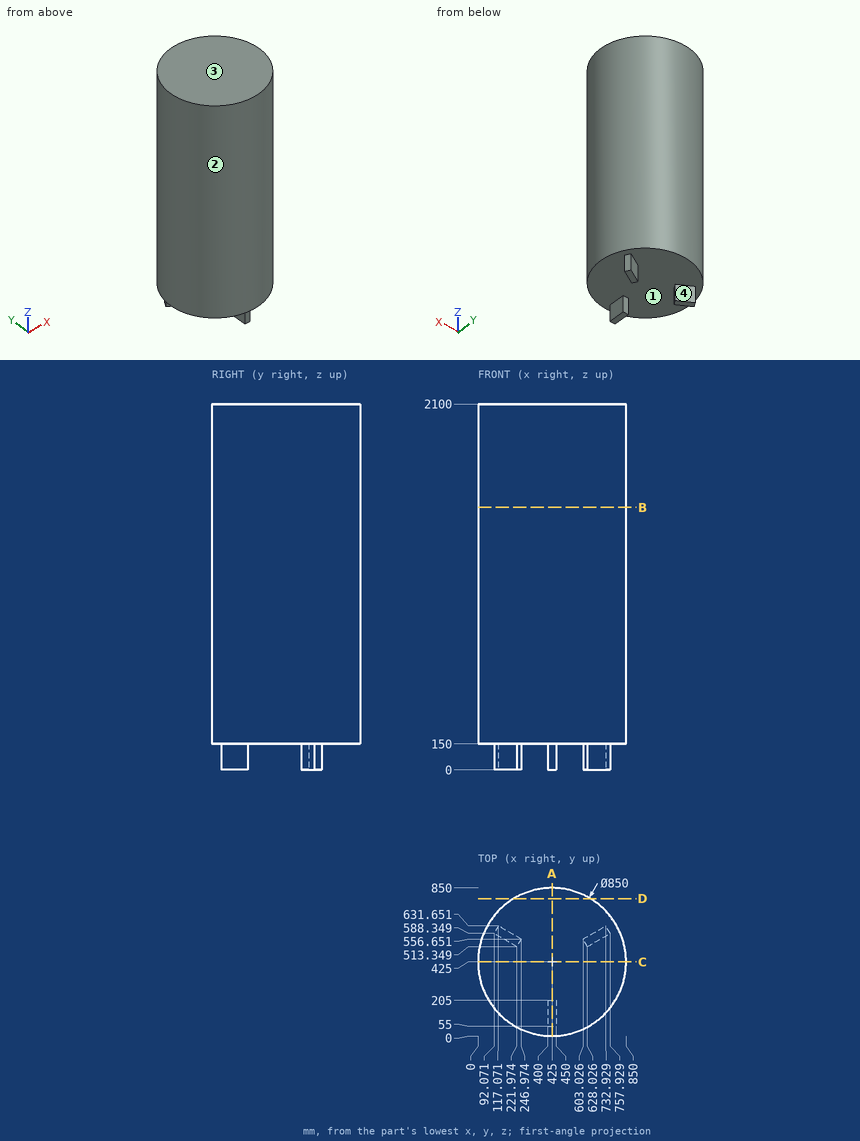
Study the drawing (mm; zero at the part's minimum x, y, z) and answer. Give positions to 0.01 mm unless a question says otherwise; leave off trailing zeros. Write each loop counter-clockwise with the first axis right and the second up, starting at its lowest first coordinate (ties: lowest second). Pieces come first, ordered by that corner, then holes.
Item 1: Section D-D, the plane y = 788.5 is taken. Write down the section's boundary in (x, z), plus the area to 3 significant figures.
Item 2: Section B-B, the plane z = 1506 is taken. Write down the section's boundary in (x, y).
Item 3: Find the intervals of material crossed by line 1 along Y through (x, z) = (432, 676.5); line 2 along Z through (x, y) = (591, 768.5); line 3 along X through (y, z) = (413, 340.5), in increasing order.
Item 4: Section C-C, the plane y = 425 is taken. Write down the section's boundary in (x, z).
Item 5: Section A-A, the plane x = 425 is taken. Write down the section's boundary in (y, z).
Item 6: Flat-ended cylindrical pins translate along their axes: P1, Ø2, axis at x = 150.5, z = 1603, coming from the -Y side (1 decimal); P2, Ø8, axis at x = 594.5, z = 339.5, coming from the +Y side; P3, Ø1, axis at x = 247.5, z = 231, coming from the -Y side. Find the tip coordinate at first contact, or state that the pin passes through.
Item 7: Determine the mould class of the marked faces 1, 2, 3 and 4 for opening direction X: released by +X, released by -X, zero draft, split by the parting line, or undercut.
Completed:
1. outline: (204.79, 150) - (645.21, 150) - (645.21, 2100) - (204.79, 2100) - close
1. area: 859,000 mm2
2. outline: circle Ø850 at (425, 425)
3. line 1: y = 0.06 to 849.94
3. line 2: z = 150 to 2100
3. line 3: x = 0.17 to 849.83
4. outline: (0, 150) - (850, 150) - (850, 2100) - (0, 2100) - close
5. outline: (0, 150) - (55, 150) - (55, 0) - (205, 0) - (205, 150) - (850, 150) - (850, 2100) - (0, 2100) - close
6. P1: stops at y = 99.7
6. P2: stops at y = 816.45
6. P3: stops at y = 38.61
7. face 1: undercut
7. face 2: split by the parting line
7. face 3: zero draft
7. face 4: undercut
